```python
from build123d import *

# Parameters (mm, degrees)
CROQUIS1_R              = 18.4
SALIENTE_EXTRUIR1_DEPTH = 26.3
CROQUIS2_R              = 1.5
CORTAR_EXTRUIR1_DEPTH   = 3
CROQUIS3_R              = 5
CORTAR_EXTRUIR2_DEPTH   = 44
CORTAR_EXTRUIR3_START   = -3
CROQUIS4_R              = 1.5
CORTAR_EXTRUIR3_DEPTH   = 3


with BuildPart() as part:
    # Croquis1 → Saliente-Extruir1 (new body)
    with BuildSketch(Plane.XY):
        Circle(CROQUIS1_R)
    extrude(amount=SALIENTE_EXTRUIR1_DEPTH)

    # Croquis2 → Cortar-Extruir1 (cut)
    with BuildSketch(Plane.XY.offset(26.3)):
        with Locations((0, 8)):
            Circle(CROQUIS2_R)
        with Locations((8, 0)):
            Circle(CROQUIS2_R)
        with Locations((0, -8)):
            Circle(CROQUIS2_R)
        with Locations((-8, 0)):
            Circle(CROQUIS2_R)
    extrude(amount=-CORTAR_EXTRUIR1_DEPTH, mode=Mode.SUBTRACT)

    # Croquis3 → Cortar-Extruir2 (cut)
    with BuildSketch(Plane.XY.offset(26.3)):
        Circle(CROQUIS3_R)
    extrude(amount=-CORTAR_EXTRUIR2_DEPTH, mode=Mode.SUBTRACT)

    # Croquis4 → Cortar-Extruir3 (cut)
    with BuildSketch(Plane(origin=(0, 0, 0), x_dir=(-1, 0, 0), z_dir=(0, 0, -1)).offset(CORTAR_EXTRUIR3_START)):
        with Locations(Location((0, 8, 0), (0, 0, 180))):
            Circle(CROQUIS4_R)
        with Locations(Location((8, 0, 0), (0, 0, 180))):
            Circle(CROQUIS4_R)
        with Locations(Location((0, -8, 0), (0, 0, 180))):
            Circle(CROQUIS4_R)
        with Locations(Location((-8, 0, 0), (0, 0, 180))):
            Circle(CROQUIS4_R)
    extrude(amount=CORTAR_EXTRUIR3_DEPTH, mode=Mode.SUBTRACT)


solid = part.part
```
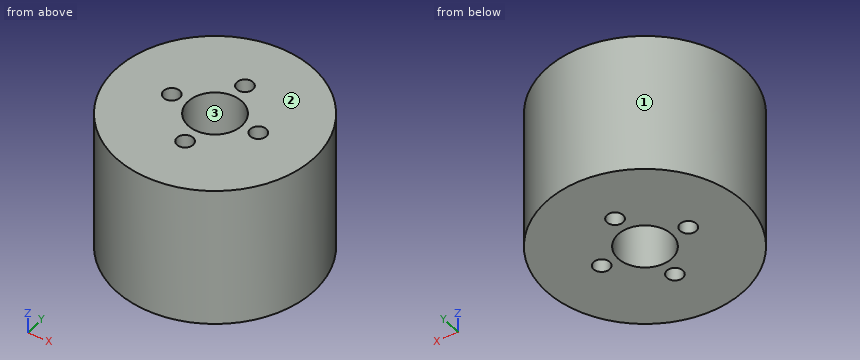
For this review, take the finished solid that the model builds, in its own axes (mm). Face numbers are marked on the shaded views. Round coordinates to 2 decimals unless told otherwise and drop trailing zeros. Write each loop counter-clockwise with the first axis right and the second up, starting at its lowest first coordinate (ties: lowest second). Pieces come first, ordered by that corner, then holes. Notation, with made-up numbers: (15, 58) -> (39, 58) arc R21 cw to (39, 87) -> close; hole circle Ø3 at (12.5, 20). An arc over 180 degrees is marked (long way). Use one line per item in the form item = value.
Q1. Consider section C-C (z = 4.75). State the section outline as (x, y) points.
Resolved:
outline = circle Ø36.8 at (0, 0); hole circle Ø10 at (0, 0)
Q2. The part is to be moulded in two halves that separate along X. For the marked faces 1, 2 and 3, say which applies: released by +X, released by -X, zero draft, split by the parting line, or undercut.
Resolved:
face_1 = split by the parting line
face_2 = zero draft
face_3 = undercut
Q3. Clearance check with flat-ended pins moving along their axes: pin 1 Ø0.9 at (x, y) = (7.5, 0.5) entering from -Z; pin 2 Ø0.9 at (x, y) = (0, -8) entering from +Z; pin 3 Ø1 at (x, z) = (5, 10.5) entering from +Y. State where each tip first meets the part, or that it passes through.
Resolved:
pin_1 = 3
pin_2 = 23.3
pin_3 = 17.84
Q4. To check wall thickness, follow probe 1 along Y at (x, z) = (0, 1); probe 2 along Y at (x, z) = (0, 12.5); probe 3 along X at (y, z) = (-8, 2.1). State the ranges of each line that lie inside material, in increasing order. Write a range as from..to.
Resolved:
probe_1 = -18.4..-9.5, -6.5..-5, 5..6.5, 9.5..18.4
probe_2 = -18.4..-5, 5..18.4
probe_3 = -16.57..-1.5, 1.5..16.57
Q5. Consider section D-D (y = 8). State the section outline as (x, z) points, then the cut area to 3 significant figures.
Resolved:
outline = (-16.57, 0) -> (-1.5, 0) -> (-1.5, 3) -> (1.5, 3) -> (1.5, 0) -> (16.57, 0) -> (16.57, 26.3) -> (1.5, 26.3) -> (1.5, 23.3) -> (-1.5, 23.3) -> (-1.5, 26.3) -> (-16.57, 26.3) -> close
area = 854 mm²
Q6. Consider section A-A (x = 0). State the section outline as (y, z) points.
Resolved:
outline = (-18.4, 0) -> (-9.5, 0) -> (-9.5, 3) -> (-6.5, 3) -> (-6.5, 0) -> (-5, 0) -> (-5, 26.3) -> (-6.5, 26.3) -> (-6.5, 23.3) -> (-9.5, 23.3) -> (-9.5, 26.3) -> (-18.4, 26.3) -> close; (5, 0) -> (6.5, 0) -> (6.5, 3) -> (9.5, 3) -> (9.5, 0) -> (18.4, 0) -> (18.4, 26.3) -> (9.5, 26.3) -> (9.5, 23.3) -> (6.5, 23.3) -> (6.5, 26.3) -> (5, 26.3) -> close
